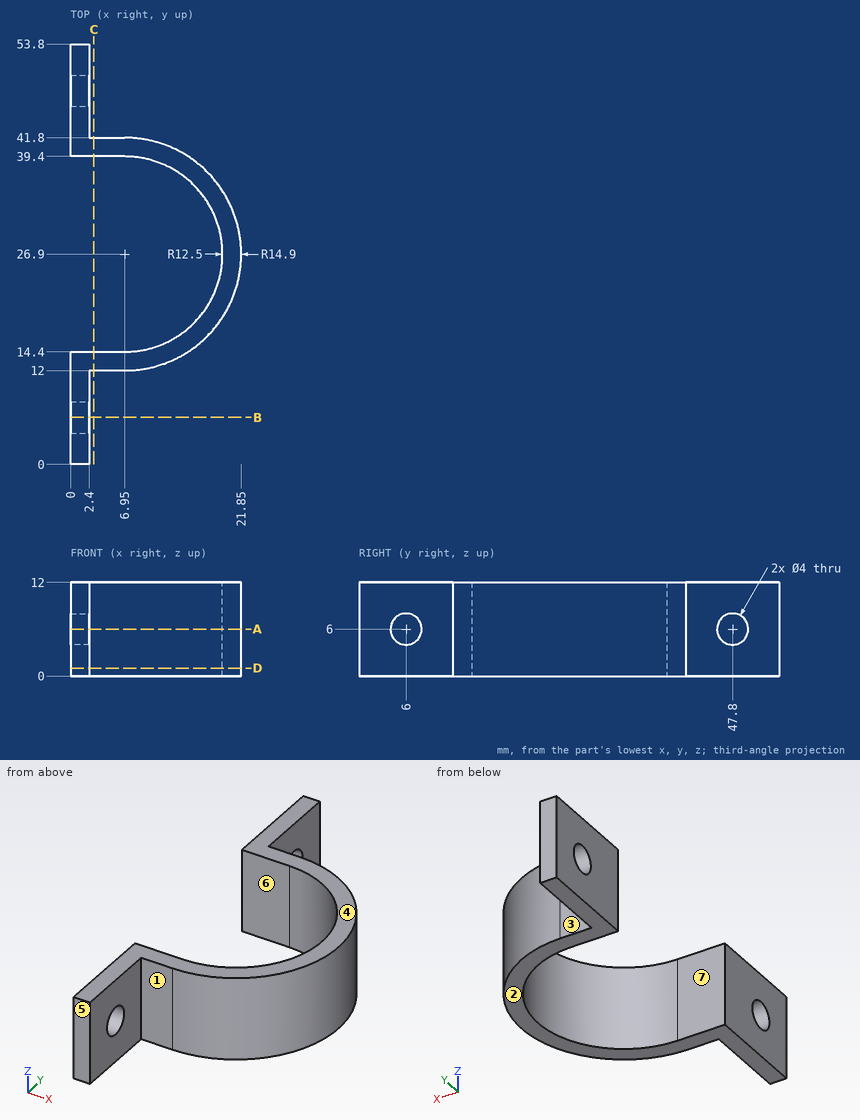
Check sheet for the drawn part. Datum: minimum x, y, z corner. Units: mm. A direction names the side the tool comes from. Round coordinates to 2 decimals unless told otherwise and drop trailing zeros. Order: outer loops, then holes, each group sorted by start corner. A loop starts at its lowest first (then second) coordinate and runs counter-clockwise, first axis right, second up.
1. Section check A-A on z = 6. Record the cut outline in (x, y), then the cut area to 3 significant figures.
Final values:
outline: (0, 0) - (2.4, 0) - (2.4, 4) - (0, 4) - close; (0, 8) - (2.4, 8) - (2.4, 12) - (6.95, 12) arc R14.9 ccw to (6.95, 41.8) - (2.4, 41.8) - (2.4, 45.8) - (0, 45.8) - (0, 39.4) - (6.95, 39.4) arc R12.5 cw to (6.95, 14.4) - (0, 14.4) - close; (0, 49.8) - (2.4, 49.8) - (2.4, 53.8) - (0, 53.8) - close
area: 175 mm2
2. Section check D-D on z = 1. Record the cut outline in (x, y), then the cut area to 3 significant figures.
Final values:
outline: (0, 0) - (2.4, 0) - (2.4, 12) - (6.95, 12) arc R14.9 ccw to (6.95, 41.8) - (2.4, 41.8) - (2.4, 53.8) - (0, 53.8) - (0, 39.4) - (6.95, 39.4) arc R12.5 cw to (6.95, 14.4) - (0, 14.4) - close
area: 194 mm2
3. Thickness scan on L1, parallel to Y at x = 1.1, z = 6; L2, parallel to Y at x = 6.75, z = 4.25; L3, parallel to X at y = 44, z = 4.5. Record the ranges inside material, lowest first.
Final values:
L1: y = 0 to 4, 8 to 14.4, 39.4 to 45.8, 49.8 to 53.8
L2: y = 12 to 14.4, 39.4 to 41.8
L3: x = 0 to 2.4
4. Access from +Z, -Z, +X, -X, +Y, -Y to the whole of each face (thin tool, end or side, straight path). Record for the marked faces 1, 2 and 3.
Final values:
face 1: +Z, -Z, +X, -Y
face 2: -Z, +X, -X, +Y, -Y
face 3: +Z, -Z, +X, +Y
5. Section check C-C on x = 3. Record the cut outline in (y, z), then the cut area to 3 significant figures.
Final values:
outline: (12, 0) - (14.4, 0) - (14.4, 12) - (12, 12) - close; (39.4, 0) - (41.8, 0) - (41.8, 12) - (39.4, 12) - close
area: 57.6 mm2
6. Go/stop test with flat-tipped pins: P1, Ø5, axis at y = 47.8, z = 6, coming from the -X side; P2, Ø5, axis at y = 44.5, z = 1.5, coming from the +X side; P3, Ø1.5, axis at x = 8, z = 8.5, coming from the -Y side; P4, Ø2.5, axis at x = 4, z = 5, coming from the +Y side. Record where each tip stops, or that it passes through.
Final values:
P1: stops at x = 0
P2: stops at x = 2.4
P3: stops at y = 12
P4: stops at y = 41.8
7. Section check B-B on y = 6. Record the cut outline in (x, z).
Final values:
outline: (0, 0) - (2.4, 0) - (2.4, 4) - (0, 4) - close; (0, 8) - (2.4, 8) - (2.4, 12) - (0, 12) - close
8. Release check for a two-part mould opening along Y. For the marked faces 4, 5, 6 and 7 record: +Y half, -Y half, draft (parallel to the pull), parting line (faces both ways), or undercut.
Final values:
face 4: draft
face 5: -Y half
face 6: undercut
face 7: undercut
